from build123d import *

# Parameters (mm, degrees)
ESQUISSE1_W             = 50.8
ESQUISSE1_H             = 254
BOSS_EXTRU_1_DEPTH      = 6.35
ESQUISSE2_W             = 127
ESQUISSE2_H             = 25.4
BOSS_EXTRU_2_DEPTH      = 6.35
CONG_1_R                = 12.7
CONG_2_R                = 2.54
ESQUISSE3_R             = 1.5
ENL_V_MAT_EXTRU_1_DEPTH = 199.481945023


with BuildPart() as part:
    # Esquisse1 → Boss.-Extru.1 (new body)
    with BuildSketch(Plane.XY):
        Rectangle(ESQUISSE1_W, ESQUISSE1_H)
    extrude(amount=BOSS_EXTRU_1_DEPTH)

    # Esquisse2 → Boss.-Extru.2 (add)
    with BuildSketch(Plane.XY.offset(6.35)):
        with Locations((88.9, -50.8)):
            Rectangle(ESQUISSE2_W, ESQUISSE2_H)
        with Locations((88.9, 50.8)):
            Rectangle(ESQUISSE2_W, ESQUISSE2_H)
    extrude(amount=-BOSS_EXTRU_2_DEPTH)

    # Congé1
    cong_1_edges = [part.edges().sort_by_distance(p)[0] for p in [
        (25.4, -63.5, 3.175),
        (25.4, -38.1, 3.175),
        (25.4, 38.1, 3.175),
        (25.4, 63.5, 3.175),
    ]]
    fillet(cong_1_edges, radius=CONG_1_R)

    # Congé2
    cong_2_edges = [part.edges().sort_by_distance(p)[0] for p in [
        (152.4, -38.1, 3.175),
        (152.4, -63.5, 3.175),
        (152.4, 63.5, 3.175),
        (152.4, 38.1, 3.175),
    ]]
    fillet(cong_2_edges, radius=CONG_2_R)

    # Esquisse3 → Enlèv. mat.-Extru.1 (cut, through all)
    with BuildSketch(Plane(origin=(0, 0, 0), x_dir=(-1, 0, 0), z_dir=(0, 0, -1))):
        with Locations((-146.05, 57.15)):
            Circle(ESQUISSE3_R)
        with Locations((-146.05, 44.45)):
            Circle(ESQUISSE3_R)
        with Locations((-146.05, -44.45)):
            Circle(ESQUISSE3_R)
        with Locations((-146.05, -57.15)):
            Circle(ESQUISSE3_R)
    extrude(amount=-ENL_V_MAT_EXTRU_1_DEPTH, mode=Mode.SUBTRACT)


solid = part.part
Model file for the job. Use its own axes, mm. A direction names the side the tool comes from. Give positions to 0.01 mm unless a question says otherwise; leave off trailing zeros. Order: outer loops, then holes, each group sorted by start corner. A loop starts at its lowest first (then second) coordinate and runs counter-clockwise, first axis right, second up. Notation, with made-up numbers: M 75,19.5 L 85,19.5 A12 ccw 85,33.5 Z; hole C 28.5,18 d7. An arc over 180 degrees is marked long. Write item = value, one per line.
Q1. Drill centre lines: line 1 (Y direction, x = 146.05, z = 3.5); line 2 (Y direction, x = 114.5, z = 2.5); line 3 (X direction, y = 75.5, z = 0.5). Where is each one in solid material? Low to high. Write a range as [from, to].
Derived:
line_1 = [-63.5, -58.65], [-55.65, -45.95], [-42.95, -38.1], [38.1, 42.95], [45.95, 55.65], [58.65, 63.5]
line_2 = [-63.5, -38.1], [38.1, 63.5]
line_3 = [-25.4, 25.42]
Q2. Two-plate mould, pull along Y, no slides. Class faces 6 (the flat face through (93, -63.5, 3)), 7 (the cylindrical face through (29.02, -34.28, 3.13)), 8 (the flat face through (23, 2, 6.35)): pulls with the +Y half, pulls with the -Y half, needs draft (parallel to the pull), parting line crosses it, or undercut.
Derived:
face_6 = pulls with the -Y half
face_7 = undercut
face_8 = needs draft
Q3. Tool access for faces 1 (the flat face through (0, 127, 3)), 2 (the flat face through (25.4, 101, 3)), 3 (the flat face through (23, 2, 0)), 4 (the flat face through (93, 38.1, 3)), 5 (the flat face through (25.4, -102, 3)): list every direction of +Z, -Z, +X, -X, +Y, -Y with a clear straight run to the whole face (end or side of a thin tool).
Derived:
face_1 = +Z, -Z, +X, -X, +Y
face_2 = +Z, -Z, +X, +Y
face_3 = -Z, +X, -X, +Y, -Y
face_4 = +Z, -Z, +X
face_5 = +Z, -Z, +X, -Y
Q4. Cut at A-A, the plane x = 62. List the corners of the cut face in (y, z).
Derived:
outline = M -63.5,0 L -38.1,0 L -38.1,6.35 L -63.5,6.35 Z; M 38.1,0 L 63.5,0 L 63.5,6.35 L 38.1,6.35 Z
Q5. Cut at B-B, the plane z = 3. List the corners of the cut face in (x, y).
Derived:
outline = M -25.4,-127 L 25.4,-127 L 25.4,-76.2 A12.7 cw 38.1,-63.5 L 149.86,-63.5 A2.54 ccw 152.4,-60.96 L 152.4,-40.64 A2.54 ccw 149.86,-38.1 L 38.1,-38.1 A12.7 cw 25.4,-25.4 L 25.4,25.4 A12.7 cw 38.1,38.1 L 149.86,38.1 A2.54 ccw 152.4,40.64 L 152.4,60.96 A2.54 ccw 149.86,63.5 L 38.1,63.5 A12.7 cw 25.4,76.2 L 25.4,127 L -25.4,127 Z; hole C 146.05,-57.15 d3; hole C 146.05,-44.45 d3; hole C 146.05,44.45 d3; hole C 146.05,57.15 d3
Q6. Cut at C-C, the plane y = 10.5. List the corners of the cut face in (x, z).
Derived:
outline = M -25.4,0 L 25.4,0 L 25.4,6.35 L -25.4,6.35 Z
Q7. Cut at D-D, the plane y = -28.5. List the corners of the cut face in (x, z).
Derived:
outline = M -25.4,0 L 25.78,0 L 25.78,6.35 L -25.4,6.35 Z
Q8. Flat gauge pins, fed straight in: pin 1 (4 mm diameter, centred on x = 146.05, y = 44.45, fed in from -Z); pin 2 (3 mm diameter, centred on x = 95.5, z = 2.5, fed in from -Y); pin 3 (1.9 mm diameter, centred on y = 106.5, z = 2, fed in from +X); pin 4 (3 mm diameter, centred on x = 91, z = 2, fed in from +Y). Where does each tip first touch, or does it go through?
Derived:
pin_1 = 0
pin_2 = -63.5
pin_3 = 25.4
pin_4 = 63.5
